Source: CAD feature listing. Evaluate the final solid. Frame: model axes, mm. A direction names the side the tool comes from. Give positions to 0.01 mm unless a question says otherwise; leave off trailing zeros. Order: outer loops, then holes, each group sorted by start corner. A loop starts at its lowest first (then second) coordinate and runs counter-clockwise, first axis right, second up.
1) First-contact query: P1, Ø6, axis at x = 55, y = -79.7, coming from the -Z side; P2, Ø8.5, axis at x = 55, y = -10.58, coming from the -Z side. Flat tips, straight axial feed; report the tip coordinate or a pass-through.
2) Section B-B, the plane y = -32.5. Return loops of the section in (x, z).
3) Draft query along X for faces 3 (the face through (53, -8, 8)), 4 (the face through (35, -44, 0)), 5 (the face through (69.43, -89.4, 6.44)). Return one class per face: released by +X, released by -X, zero draft, split by the parting line, or undercut.
4) Access query for faces 1 (the face through (51.59, -10.43, 3.48)), 2 (the face through (26, -10.785, 6)). Directions: +Z, -Z, +X, -X, +Y, -Y. A direction counts if a zero-diameter tool reaches every point of the face in a straight line with its end or side. Return the directions, or none.
5) Section C-C, the plane x = 38.5. Return loops of the section in (y, z) (3 decimals), plus the area to 3 significant figures.
6) Material intervals for line 1 (Y direction, x = 29.5, z = 8.75) (3 decimals); line 2 (Y direction, x = 55, z = 9.5) (3 decimals); line 3 (Y direction, x = 51.5, z = 5) (3 decimals), sorted ascending.
7) Section D-D, the plane z = 10.5. Return loops of the section in (x, y) (3 decimals), plus the area to 3 significant figures.
8) Section A-A, the plane x = 55. Return loops of the section in (y, z) (3 decimals).
```python
from build123d import *

# Parameters (mm, degrees)
SKETCH1_W                                        = 70
SKETCH1_H                                        = 90
BOSS_EXTRUDE1_DEPTH                              = 12.7
CSK_FOR_1_4_FLAT_HEAD_MACHINE_SCREW1_D           = 6.5278
CSK_FOR_1_4_FLAT_HEAD_MACHINE_SCREW1_CSINK_D     = 12.8778
CSK_FOR_1_4_FLAT_HEAD_MACHINE_SCREW1_CSINK_ANGLE = 82
FILLET1_R                                        = 2
CUT_EXTRUDE1_DEPTH                               = 115.72266559


with BuildPart() as part:
    # Sketch1 → Boss-Extrude1 (new body)
    with BuildSketch(Plane.XY):
        with Locations((35, -45)):
            Rectangle(SKETCH1_W, SKETCH1_H)
        Polygon((55, -29.025), (61.45, -29.025), (61.45, -60.975), (55, -60.975), (48.55, -60.975), (48.55, -29.025), align=None, mode=Mode.SUBTRACT)
    extrude(amount=BOSS_EXTRUDE1_DEPTH)

    # CSK for 1/4 Flat Head Machine Screw1 (through all)
    with Locations(Plane(origin=(0, 0, 0), x_dir=(-1, 0, 0), z_dir=(0, 0, -1))):
        with Locations((-55, -10.579610023), (-55, -79.699610023)):
            CounterSinkHole(CSK_FOR_1_4_FLAT_HEAD_MACHINE_SCREW1_D / 2, CSK_FOR_1_4_FLAT_HEAD_MACHINE_SCREW1_CSINK_D / 2, counter_sink_angle=CSK_FOR_1_4_FLAT_HEAD_MACHINE_SCREW1_CSINK_ANGLE)

    # Fillet1
    fillet1_edges = [part.edges().sort_by_distance(p)[0] for p in [
        (0, 0, 6.35),
        (70, 0, 6.35),
        (70, -90, 6.35),
        (0, -90, 6.35),
    ]]
    fillet(fillet1_edges, radius=FILLET1_R)

    # Sketch7 → Cut-Extrude1 (cut, through all)
    with BuildSketch(Plane(origin=(0, 0, 0), x_dir=(-1, 0, 0), z_dir=(0, 0, -1))):
        with BuildLine():
            Line((-41.687469931, -85.815), (-11.687469931, -85.815))
            ThreePointArc((-11.687469931, -85.815), (-8.387469931, -82.515), (-11.687469931, -79.215))
            Line((-11.687469931, -79.215), (-41.687469931, -79.215))
            ThreePointArc((-41.687469931, -79.215), (-44.987469931, -82.515), (-41.687469931, -85.815))
        make_face()
        with BuildLine():
            Line((-11.687469931, -10.785), (-41.687469931, -10.785))
            ThreePointArc((-41.687469931, -10.785), (-44.987469931, -7.485), (-41.687469931, -4.185))
            Line((-41.687469931, -4.185), (-11.687469931, -4.185))
            ThreePointArc((-11.687469931, -4.185), (-8.387469931, -7.485), (-11.687469931, -10.785))
        make_face()
    extrude(amount=-CUT_EXTRUDE1_DEPTH, mode=Mode.SUBTRACT)


solid = part.part
```
From the geometry:
1. P1: passes through
1. P2: stops at z = 2.52
2. outline: (0, 0) - (48.55, 0) - (48.55, 12.7) - (0, 12.7) - close; (61.45, 0) - (70, 0) - (70, 12.7) - (61.45, 12.7) - close
3. face 3: undercut
3. face 4: zero draft
3. face 5: released by +X
4. face 1: -Z
4. face 2: +Z, -Z
5. outline: (-90, 0) - (-85.815, 0) - (-85.815, 12.7) - (-90, 12.7) - close; (-79.215, 0) - (-10.785, 0) - (-10.785, 12.7) - (-79.215, 12.7) - close; (-4.185, 0) - (0, 0) - (0, 12.7) - (-4.185, 12.7) - close
5. area: 975 mm2
6. line 1: y = -90 to -85.815, -79.215 to -10.785, -4.185 to 0
6. line 2: y = -90 to -82.964, -76.436 to -60.975, -29.025 to -13.844, -7.316 to 0
6. line 3: y = -90 to -60.975, -29.025 to 0
7. outline: (0, -88) arc R2 ccw to (2, -90) - (68, -90) arc R2 ccw to (70, -88) - (70, -2) arc R2 ccw to (68, 0) - (2, 0) arc R2 ccw to (0, -2) - close; hole (11.687, -85.815) - (41.687, -85.815) arc R3.3 ccw to (41.687, -79.215) - (11.687, -79.215) arc R3.3 ccw to start; hole (11.687, -10.785) - (41.687, -10.785) arc R3.3 ccw to (41.687, -4.185) - (11.687, -4.185) arc R3.3 ccw to start; hole (48.55, -60.975) - (61.45, -60.975) - (61.45, -29.025) - (48.55, -29.025) - close; hole circle Ø6.528 at (55, -79.7); hole circle Ø6.528 at (55, -10.58)
7. area: 5,350 mm2
8. outline: (-90, 0) - (-86.139, 0) - (-82.964, 3.652) - (-82.964, 12.7) - (-90, 12.7) - close; (-76.436, 3.652) - (-73.261, 0) - (-60.975, 0) - (-60.975, 12.7) - (-76.436, 12.7) - close; (-29.025, 0) - (-17.019, 0) - (-13.844, 3.652) - (-13.844, 12.7) - (-29.025, 12.7) - close; (-7.316, 3.652) - (-4.141, 0) - (0, 0) - (0, 12.7) - (-7.316, 12.7) - close
